from build123d import *

# Parameters (mm, degrees)
SKETCH1_W           = 34
SKETCH1_H           = 30
SKETCH1_R           = 2.25
BOSS_EXTRUDE1_DEPTH = 5
SKETCH2_W           = 5
SKETCH2_H           = 30
BOSS_EXTRUDE2_DEPTH = 15
SKETCH4_W           = 5
SKETCH4_H           = 30
BOSS_EXTRUDE3_DEPTH = 25
SKETCH5_R           = 2.5
CUT_EXTRUDE1_DEPTH  = 25


with BuildPart() as part:
    # Sketch1 → Boss-Extrude1 (new body)
    with BuildSketch(Plane.XY):
        with Locations((17, 15)):
            Rectangle(SKETCH1_W, SKETCH1_H)
        with Locations((4.75, 25.25)):
            Circle(SKETCH1_R, mode=Mode.SUBTRACT)
        with Locations((29.25, 25.25)):
            Circle(SKETCH1_R, mode=Mode.SUBTRACT)
        with Locations((29.25, 4.75)):
            Circle(SKETCH1_R, mode=Mode.SUBTRACT)
        with Locations((4.75, 4.75)):
            Circle(SKETCH1_R, mode=Mode.SUBTRACT)
    extrude(amount=BOSS_EXTRUDE1_DEPTH)

    # Sketch2 → Boss-Extrude2 (add)
    with BuildSketch(Plane.ZY):
        with Locations((2.5, 15)):
            Rectangle(SKETCH2_W, SKETCH2_H)
    extrude(amount=BOSS_EXTRUDE2_DEPTH)

    # Sketch4 → Boss-Extrude3 (add)
    with BuildSketch(Plane.XY.offset(5)):
        with Locations((-12.5, 15)):
            Rectangle(SKETCH4_W, SKETCH4_H)
    extrude(amount=BOSS_EXTRUDE3_DEPTH)

    # Sketch5 → Cut-Extrude1 (cut)
    with BuildSketch(Plane(origin=(-10, 0, 0), x_dir=(0, 0, -1), z_dir=(1, 0, 0))):
        with Locations((-24, 15)):
            Circle(SKETCH5_R)
        with Locations((-10, 15)):
            Circle(SKETCH5_R)
    extrude(amount=-CUT_EXTRUDE1_DEPTH, mode=Mode.SUBTRACT)


solid = part.part
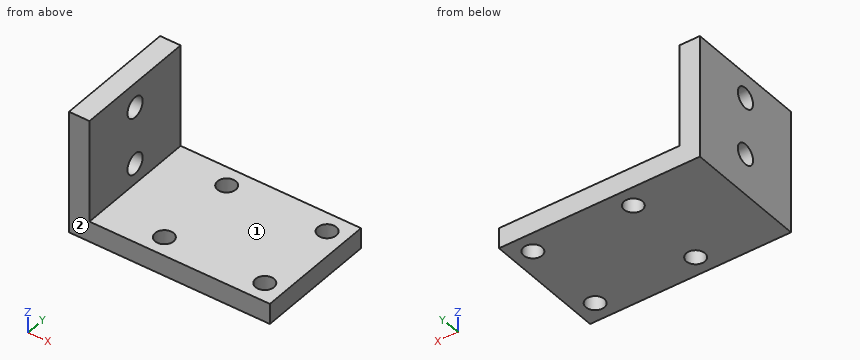
Part model, mm, in its own coordinate system. Face numbers are marked on the shaded views. A direction names the side the tool comes from. Give positions to 0.01 mm unless a question says otherwise; leave off trailing zeros. Write each loop counter-clockwise with the first axis right and the second up, starting at its lowest first coordinate (ties: lowest second). Pieces come first, ordered by that corner, then holes.
1) Cut at D-D on x = -11. Write the cut outline in (y, z).
Resolved:
outline: (0, 0) - (30, 0) - (30, 30) - (0, 30) - close; hole circle Ø5 at (15, 10); hole circle Ø5 at (15, 24)
2) Cut at A-A on z = 24. Write the cut outline in (x, y).
Resolved:
outline: (-15, 0) - (-10, 0) - (-10, 12.5) - (-15, 12.5) - close; (-15, 17.5) - (-10, 17.5) - (-10, 30) - (-15, 30) - close
3) Cut at C-C on y = 15. Write the cut outline in (x, z), then the cut area to 3 significant figures.
Resolved:
outline: (-15, 0) - (34, 0) - (34, 5) - (-10, 5) - (-10, 7.5) - (-15, 7.5) - close; (-15, 12.5) - (-10, 12.5) - (-10, 21.5) - (-15, 21.5) - close; (-15, 26.5) - (-10, 26.5) - (-10, 30) - (-15, 30) - close
area: 320 mm2
4) Cut at B-B on x = 29.25. Write the cut outline in (y, z).
Resolved:
outline: (0, 0) - (2.5, 0) - (2.5, 5) - (0, 5) - close; (7, 0) - (23, 0) - (23, 5) - (7, 5) - close; (27.5, 0) - (30, 0) - (30, 5) - (27.5, 5) - close
5) Probe L1, parallel to Y at x = -11, z = 24; L2, parallel to Y at x = 29.25, z = 2.35; L3, parallel to Y at x = 6, z = 4. List the from-to ranges inside material, lowest first.
Resolved:
L1: y = 0 to 12.5, 17.5 to 30
L2: y = 0 to 2.5, 7 to 23, 27.5 to 30
L3: y = 0 to 2.88, 6.62 to 23.38, 27.12 to 30
6) Pin check, flat tips, straight feed: pin 1 (3 mm diameter, centred on y = 15, z = 10, fed in from -X); pin 2 (6 mm diameter, centred on x = 29.25, y = 4.75, fed in from +Z); pin 3 (8 mm diameter, centred on y = 14.5, z = 22.5, fed in from +X). Stop position of each tip, or through.
Resolved:
pin 1: passes through
pin 2: stops at z = 5
pin 3: stops at x = -10
7) Which spindle directions (+Z, -Z, +X, -X, +Y, -Y) get a long thin tool onto all of the face, cutting with end or side? Do the marked faces 1 and 2. Say none if no direction does.
Resolved:
face 1: +Z, +X, +Y, -Y
face 2: +Z, -Z, +X, -X, -Y
